Autodesk Inventor part; units mm, degrees
ref_plane "YZ Plane" through (0, 0, 0) normal (1, 0, 0) x (0, 1, 0)
ref_plane "XZ Plane" through (0, 0, 0) normal (0, 1, 0) x (-1, 0, 0)
ref_plane "XY Plane" through (0, 0, 0) normal (0, 0, 1) x (1, 0, 0)
sketch "Sketch_1" plane through (0, 0, 0) normal (0, 0, 1) x (1, 0, 0)
  line L0 (130, 0) -> (0, 0)
  line L1 (0, 0) -> (0, 6.5)
  line L2 (0, 6.5) -> (0.5, 7)
  line L3 (0.5, 7) -> (20, 7)
  line L4 (20, 7) -> (20, 9.5)
  line L5 (20, 9.5) -> (20.5, 10)
  line L6 (20.5, 10) -> (29.5, 10)
  line L7 (29.5, 10) -> (30, 9.5)
  line L8 (30, 9.5) -> (30, 8.5)
  line L9 (30, 8.5) -> (109.5, 8.5)
  line L10 (109.5, 8.5) -> (110, 8)
  line L11 (110, 8) -> (110, 6)
  line L12 (110, 6) -> (129.5, 6)
  line L13 (129.5, 6) -> (130, 5.5)
  line L14 (130, 5.5) -> (130, 0)
  line L15 (130, 0) -> (0, 0)
revolve "Revolution1" add sketch "Sketch_1" angle 360 about axis through (130, 0, 0) along (1, 0, 0)
sketch "Sketch_2" plane through (0, 0, 0) normal (0, 0, 1) x (1, 0, 0)
  line L0 (50, 0) -> (-50, 0)
  line L1 (18.5, 6.7) -> (20, 6.7)
  line L2 (20, 6.7) -> (20, 20.7)
  line L3 (20, 20.7) -> (18.5, 20.7)
  line L4 (18.5, 20.7) -> (18.5, 6.7)
revolve "Revolution2" cut sketch "Sketch_2" angle 360 about axis through (50, 0, 0) along (1, 0, 0)
sketch "Sketch_3" plane through (0, 0, 0) normal (0, 0, 1) x (1, 0, 0)
  line L0 (260, 0) -> (-260, 0)
  line L1 (30, 8.2) -> (31.5, 8.2)
  line L2 (31.5, 8.2) -> (31.5, 22.2)
  line L3 (31.5, 22.2) -> (30, 22.2)
  line L4 (30, 22.2) -> (30, 8.2)
revolve "Revolution3" cut sketch "Sketch_3" angle 360 about axis through (260, 0, 0) along (1, 0, 0)
sketch "Sketch_4" plane through (0, 0, 0) normal (0, 0, 1) x (1, 0, 0)
  line L0 (50, 0) -> (-50, 0)
  line L1 (110, 5.7) -> (111.5, 5.7)
  line L2 (111.5, 5.7) -> (111.5, 19.7)
  line L3 (111.5, 19.7) -> (110, 19.7)
  line L4 (110, 19.7) -> (110, 5.7)
revolve "Revolution4" cut sketch "Sketch_4" angle 360 about axis through (50, 0, 0) along (1, 0, 0)
sketch "Sketch_15" plane through (0, 8.5, 0) normal (0, 1, 0) x (1, 0, 0)
  arc A0 (34.5, 2.5) -> (34.5, -2.5) centre (34.5, 0) ccw
  line L0 (34.5, -2.5) -> (49.5, -2.5)
  arc A1 (49.5, -2.5) -> (49.5, 2.5) centre (49.5, 0) ccw
  line L1 (49.5, 2.5) -> (34.5, 2.5)
extrude "Extrusion1" cut sketch "Sketch_15" against normal blind 3
properties part number "KZFC17-130-T10-P14-LA20-Q12-LB20-KC58-HC20_b"
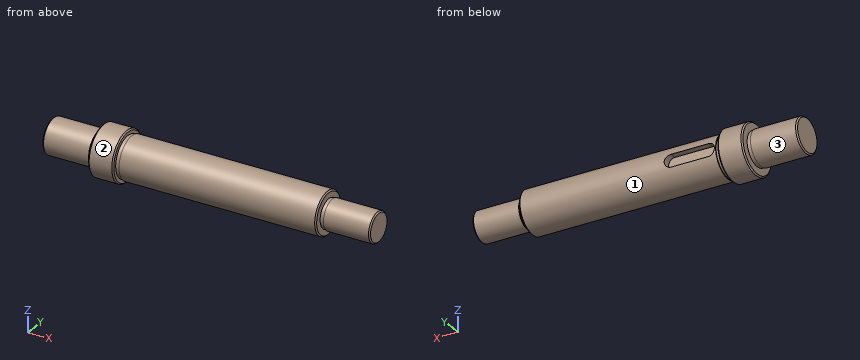
The listing builds one solid part. Answer for the finished solid, in the listing's coordinates (mm). Face numbers are marked on the shaded views. A direction names the side the tool comes from. Give positions to 0.01 mm unless a question says otherwise; leave off trailing zeros. Loops run counter-clockwise (first coordinate to the right, second up) from the corner with the lowest first, then second, coordinate; pieces in that order, holes last. Notation, with made-up numbers: (51, 61) - (91, 61) arc R15 ccw to (91, 69) - close; hole circle Ø7 at (56.5, -1). An arc over 180 degrees is marked (long way). Return JSON: item names as keys, results as strings. Group by question number.
1. Find section A-A (x = 75.5). Write down the section's boundary in (y, z).
2. Given pin 1 Ø1 at (x, y) = (17.5, 4) entering from +Z; pin 2 Ø0.8 at (x, y) = (42.5, 7.5) entering from +Z; pin 3 Ø6 at (x, y) = (68, -8) entering from -Z, each flat-ended and moving along its own axis, determine where each tip first touches the part or whether it passes through.
3. Which of the six approach directions +Z, -Z, +X, -X, +Y, -Y give full straight-line access (tool end or side, diameter ignored) to the marked faces 1, 2 and 3?
4. Straight lines are drawn through the part: line 1 (Z direction, x = 10, y = -0.5); line 2 (X direction, y = 4.75, z = -5); line 3 (X direction, y = 2, z = 6). For each, find the intervals that lie inside material, in ascending order. Write a range as [from, to].
Verdict:
{
 "1": {"outline": "circle Ø17 at (0, 0)"},
 "2": {"pin 1": "stops at z = 6.06", "pin 2": "stops at z = 4.67", "pin 3": "stops at z = -6.87"},
 "3": {"face 1": "+X", "face 2": "+X, -X", "face 3": "-X"},
 "4": {"line 1": "z = [-6.98, 6.98]", "line 2": "x = [0.4, 18.5], [20, 110]", "line 3": "x = [0, 110]"}
}
